```python
from build123d import *

# Parameters (mm, degrees)
SKETCH1_R           = 11.5062
BOSS_EXTRUDE2_DEPTH = 4.7625
BOSS_EXTRUDE3_DEPTH = 3.175
FILLET1_R           = 3.175
CHAMFER1_SIZE       = 0.889


with BuildPart() as part:
    # Sketch1 → Boss-Extrude2 (new, symmetric)
    with BuildSketch(Plane.XY):
        with BuildLine():
            ThreePointArc((14.563243761, 1.857300354), (-4.811299793, 13.870437187), (-12.585193267, -7.559797873))
            ThreePointArc((-12.585193267, -7.559797873), (4.811299793, -13.870437187), (14.563243761, 1.857300354))
        make_face()
        with Locations(Location((0, 0, 0), (0, 0, 180))):
            Circle(SKETCH1_R, mode=Mode.SUBTRACT)
    extrude(amount=BOSS_EXTRUDE2_DEPTH, both=True)

    # Sketch1_4 → Boss-Extrude3 (add, symmetric)
    with BuildSketch(Plane.XY):
        with BuildLine():
            ThreePointArc((-12.585193267, -7.559797873), (-10.89585042, -11.492870345), (-10.31875, -15.734319794))
            Line((-10.31875, -15.734319794), (-10.31875, -43.039319794))
            Line((-10.31875, -43.039319794), (10.31875, -43.039319794))
            Line((10.31875, -43.039319794), (10.31875, -29.747797869))
            Line((10.31875, -29.747797869), (22.874796512, -45.668948499))
            Line((22.874796512, -45.668948499), (39.079387582, -32.889369691))
            Line((39.079387582, -32.889369691), (17.84562587, -5.964818374))
            ThreePointArc((17.84562587, -5.964818374), (15.672287957, -2.277062873), (14.563243761, 1.857300354))
            ThreePointArc((14.563243761, 1.857300354), (4.811299793, -13.870437187), (-12.585193267, -7.559797873))
        make_face()
        with BuildLine():
            ThreePointArc((5.55625, -32.720569794), (0, -38.276819794), (-5.55625, -32.720569794))
            Line((-5.55625, -32.720569794), (-5.55625, -27.958069794))
            ThreePointArc((-5.55625, -27.958069794), (0, -22.401819794), (5.55625, -27.958069794))
            Line((5.55625, -27.958069794), (5.55625, -32.720569794))
        make_face(mode=Mode.SUBTRACT)
        with BuildLine():
            ThreePointArc((28.950077162, -27.736207727), (28.027958476, -35.539638078), (20.224528124, -34.617519392))
            Line((20.224528124, -34.617519392), (17.275394553, -30.877998376))
            ThreePointArc((17.275394553, -30.877998376), (18.197513239, -23.074568025), (26.000943591, -23.996686711))
            Line((26.000943591, -23.996686711), (28.950077162, -27.736207727))
        make_face(mode=Mode.SUBTRACT)
    extrude(amount=BOSS_EXTRUDE3_DEPTH, both=True)

    # Fillet1
    fillet1_edges = [part.edges().sort_by_distance(p)[0] for p in [
        (-10.31875, -43.039319794, 0),
        (10.31875, -43.039319794, 0),
        (10.31875, -29.747797869, 0),
        (22.874796512, -45.668948499, 0),
        (39.079387582, -32.889369691, 0),
    ]]
    fillet(fillet1_edges, radius=FILLET1_R)

    # Chamfer1
    chamfer1_edges = [part.edges().sort_by_distance(p)[0] for p in [
        (11.5062, 0, -4.7625),
        (11.5062, 0, 4.7625),
    ]]
    chamfer(chamfer1_edges, length=CHAMFER1_SIZE)


solid = part.part
```
Model file for the job. Use its own axes, mm. A direction names the side the tool comes from. Coordinates: 2 decimals unless noted, no trailing zeros. Loops run counter-clockwise (first coordinate to the right, second up) from the corner with the lowest first, then second, coordinate; pieces in that order, holes last. Notation, with made-up numbers: (-23.5, 77) - (29.5, 77) arc R12 ccw to (29.5, 91) - close; hole circle Ø10 at (22.25, 48). An arc over 180 degrees is marked (long way). Answer as a JSON object with one key per item and string values. Group by question number.
(1) Tool access for faces 4 (the face through (-9.4, -42.1, 0)), 5 (the face through (0.122, -38.275, 0.044)), 6 (the face through (18.41, -40.01, 0.04)): list every direction of +Z, -Z, +X, -X, +Y, -Y with a clear straight run to the whole face (end or side of a thin tool).
(2) Cut at B-B (z = -1.5). State how many separate pieces and enclosed holes the cut face has, then the cut area to 3 significant figures.
(3) Probe line 1 along Y through (x, z) = (0, -1.45); line 2 along Y through (x, z) = (5, 1.5); line 3 along X through (y, z) = (3, -4). List the from-to ranges inside material, lowest first.
(4) Flat gauge pins, fed straight in: pin 1 (20.5 mm diameter, centred on x = 0, y = 0, fed in from +Z); pin 2 (6 mm diameter, centred on x = 17, y = -38, fed in from +Z) (3 decimals); pin 3 (2 mm diameter, centred on x = 27.5, z = 2, fed in from +Y); pin 4 (23 mm diameter, centred on x = 4, y = -16.5, fed in from -Z). Where does each tip first touch, or does it go through?
(5) Two-plate mould, pull along Y, no slides. Class faces 1 (the face through (-10, -8, -4.762)), 2 (the face through (5.556, -30, 0)), 3 (the face through (0, -43.039, 0)): released by +Y, released by -Y, zero draft, split by the parting line, or undercut.
(6) Cut at A-A (x = 0). Give the cut face in (y, z) (1 decimal), then the cut area to 3 significant figures.
(7) Cut at D-D (y = -29). Give the cut face in (x, z) (3 decimals), then the cut area to 3 significant figures.
Geometry says:
{
 "1": {"face 4": "+Z, -Z, -X, -Y", "face 5": "+Z, -Z", "face 6": "+Z, -Z, -Y"},
 "2": {"separate pieces": "1", "enclosed holes": "3", "area": "1,240 mm^2"},
 "3": {"line 1": "y = -43.04 to -38.28, -22.4 to -11.51, 11.51 to 14.68", "line 2": "y = -43.04 to -35.14, -25.53 to -10.36, 10.36 to 13.8", "line 3": "x = -14.37 to -11.24, 11.24 to 14.37"},
 "4": {"pin 1": "passes through", "pin 2": "stops at z = 3.175", "pin 3": "stops at y = -16.94", "pin 4": "stops at z = -4.76"},
 "5": {"face 1": "zero draft", "face 2": "undercut", "face 3": "released by -Y"},
 "6": {"outline": "(-43, -3.2) - (-38.3, -3.2) - (-38.3, 3.2) - (-43, 3.2) - close; (-22.4, -3.2) - (-14.7, -3.2) - (-14.7, -4.8) - (-12.4, -4.8) - (-11.5, -3.9) - (-11.5, 3.9) - (-12.4, 4.8) - (-14.7, 4.8) - (-14.7, 3.2) - (-22.4, 3.2) - close; (11.5, -3.9) - (12.4, -4.8) - (14.7, -4.8) - (14.7, 4.8) - (12.4, 4.8) - (11.5, 3.9) - close", "area": "138 mm^2"},
 "7": {"outline": "(-10.319, -3.175) - (-5.556, -3.175) - (-5.556, 3.175) - (-10.319, 3.175) - close; (5.556, -3.175) - (16.306, -3.175) - (16.306, 3.175) - (5.556, 3.175) - close; (29.699, -3.175) - (36.012, -3.175) - (36.012, 3.175) - (29.699, 3.175) - close", "area": "139 mm^2"}
}
